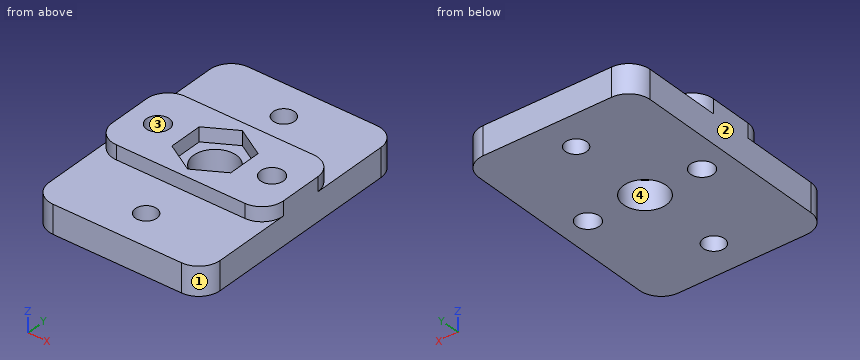
```python
from build123d import *

# Parameters (mm, degrees)
SKETCH_W          = 24
SKETCH_H          = 34
SKETCH_R          = 1.5
SKETCH_R_2        = 3
PAD_DEPTH         = 4
SKETCH001_W       = 24
SKETCH001_H       = 12
PAD001_DEPTH      = 2
SKETCH002_R       = 1.6
POCKET_DEPTH      = 4.001
POCKET_DEPTH_BACK = -2.001
FILLET_R          = 3


with BuildPart() as part:
    # Sketch → Pad (new body)
    with BuildSketch(Plane.XY):
        Rectangle(SKETCH_W, SKETCH_H)
        with Locations((0, 12)):
            Circle(SKETCH_R, mode=Mode.SUBTRACT)
        with Locations((0, -12)):
            Circle(SKETCH_R, mode=Mode.SUBTRACT)
        Circle(SKETCH_R_2, mode=Mode.SUBTRACT)
    extrude(amount=-PAD_DEPTH)

    # Sketch001 → Pad001 (join)
    with BuildSketch(Plane.XY):
        Rectangle(SKETCH001_W, SKETCH001_H)
        Polygon((4.125, -2.38157), (4.125, 2.38157), (0, 4.76314), (-4.125, 2.38157), (-4.125, -2.38157), (0, -4.76314), align=None, mode=Mode.SUBTRACT)
    extrude(amount=PAD001_DEPTH)

    # Sketch002 → Pocket (cut, two sides)
    with BuildSketch(Plane.XY) as pocket_sk:
        with Locations((-8, 0)):
            Circle(SKETCH002_R)
        with Locations((8, 0)):
            Circle(SKETCH002_R)
    extrude(amount=-POCKET_DEPTH, mode=Mode.SUBTRACT)
    extrude(pocket_sk.sketch, amount=-POCKET_DEPTH_BACK, mode=Mode.SUBTRACT)

    # Fillet
    fillet_edges = [part.edges().sort_by_distance(p)[0] for p in [
        (-12, -17, -2),
        (12, -17, -2),
        (12, -6, 1),
        (-12, -6, 1),
        (-12, 6, 1),
        (12, 6, 1),
        (12, 17, -2),
        (-12, 17, -2),
    ]]
    fillet(fillet_edges, radius=FILLET_R)


solid = part.part
```
The listing builds one solid part. Answer for the finished solid, in the listing's coordinates (mm). Face numbers are marked on the shaded views. Give positions to 0.01 mm unless a question says otherwise; leave off trailing zeros. Write each loop counter-clockwise with the first axis right and the second up, starting at its lowest first coordinate (ties: lowest second). Pieces come first, ordered by that corner, then holes. Notation, with made-up numbers: (45.5, 31.5) -> (55.5, 31.5) arc R25 ccw to (55.5, 47.5) -> close; hole circle Ø3 at (-17, -26). An arc over 180 degrees is marked (long way). Use one line per item in the form item = value.
1) Straight lines are drawn through the part: probe 1 along Y at (x, z) = (0, -1.9); probe 2 along Y at (x, z) = (-1.25, -2.5); probe 3 along Y at (x, z) = (8, -0.8). For each, find the intervals that lie inside material, in ascending order.
Result:
probe_1 = -17 to -13.5, -10.5 to -3, 3 to 10.5, 13.5 to 17
probe_2 = -17 to -12.83, -11.17 to -2.73, 2.73 to 11.17, 12.83 to 17
probe_3 = -17 to -1.6, 1.6 to 17
2) Section C-C on x = -8 is taken. Write down the section's boundary in (y, z), plus the area to 3 significant figures.
Result:
outline = (-17, -4) -> (-1.6, -4) -> (-1.6, 2) -> (-6, 2) -> (-6, 0) -> (-17, 0) -> close; (1.6, -4) -> (17, -4) -> (17, 0) -> (6, 0) -> (6, 2) -> (1.6, 2) -> close
area = 141 mm²
3) For a pull along Y with two mould halves and no side action, classify the marked faces 1, 2, 3 and 4 as +Y half, -Y half, draft (parallel to the pull), parting line (faces both ways), or undercut.
Result:
face_1 = -Y half
face_2 = draft
face_3 = undercut
face_4 = undercut
4) Section A-A on y = 0 is taken. Write down the section's boundary in (x, z) (3 decimals), plus the area to 3 significant figures.
Result:
outline = (-12, -4) -> (-9.6, -4) -> (-9.6, 2) -> (-12, 2) -> close; (-6.4, -4) -> (-3, -4) -> (-3, 0) -> (-4.125, 0) -> (-4.125, 2) -> (-6.4, 2) -> close; (3, -4) -> (6.4, -4) -> (6.4, 2) -> (4.125, 2) -> (4.125, 0) -> (3, 0) -> close; (9.6, -4) -> (12, -4) -> (12, 2) -> (9.6, 2) -> close
area = 65.1 mm²
5) Section B-B on y = -12 is taken. Write down the section's boundary in (x, z), plus the area to 3 significant figures.
Result:
outline = (-12, -4) -> (-1.5, -4) -> (-1.5, 0) -> (-12, 0) -> close; (1.5, -4) -> (12, -4) -> (12, 0) -> (1.5, 0) -> close
area = 84.0 mm²
6) Each of these flat-tipped pins is pushed along its axis until it touches: P1, Ø2.5, axis at x = 0, y = -12, coming from the -Z side (3 decimals); P2, Ø5, axis at x = 0, y = 12, coming from the +Z side; P3, Ø1.6, axis at x = 1, z = 1, coming from the +Y side. Where does it stop, or does it pass through?
Result:
P1 = through
P2 = 0
P3 = 6
7) Section D-D on z = -0.55 is taken. Write down the section's boundary in (x, y).
Result:
outline = (-12, -14) arc R3 ccw to (-9, -17) -> (9, -17) arc R3 ccw to (12, -14) -> (12, 14) arc R3 ccw to (9, 17) -> (-9, 17) arc R3 ccw to (-12, 14) -> close; hole circle Ø3.2 at (-8, 0); hole circle Ø6 at (0, 0); hole circle Ø3 at (0, -12); hole circle Ø3 at (0, 12); hole circle Ø3.2 at (8, 0)
